from build123d import *

# Parameters (mm, degrees)
EXTRUDE_1_DEPTH      = 40
FILLET_1_R           = 8
SKETCH_9_R           = 6
CUT_EXTRUDE_7_DEPTH  = 172.172427686
SKETCH_10_R          = 6
CUT_EXTRUDE_14_DEPTH = 172.172427686


with BuildPart() as part:
    # 草图8 → 凸台-拉伸1 (new, symmetric)
    with BuildSketch(Plane.XY):
        Polygon((0, 0), (140, 0), (140, 12), (12, 12), (12, 90), (0, 90), align=None)
    extrude(amount=EXTRUDE_1_DEPTH, both=True)

    # 圆角1
    fillet_1_edges = [part.edges().sort_by_distance(p)[0] for p in [
        (76, 12, 40),
        (12, 51, -40),
    ]]
    fillet(fillet_1_edges, radius=FILLET_1_R)

    # 草图9 → 切除-拉伸7 (cut, through all)
    with BuildSketch(Plane(origin=(0, 0, 0), x_dir=(1, 0, 0), z_dir=(0, 1, 0))):
        with Locations(Location((40, 6, 0), (0, 0, 90))):
            Circle(SKETCH_9_R)
    extrude(amount=CUT_EXTRUDE_7_DEPTH, mode=Mode.SUBTRACT)

    # 草图10 → 切除-拉伸14 (cut, through all)
    with BuildSketch(Plane(origin=(0, 0, 0), x_dir=(1, 0, 0), z_dir=(0, 1, 0))):
        with Locations(Location((120, 6, 0), (0, 0, 90))):
            Circle(SKETCH_10_R)
    extrude(amount=CUT_EXTRUDE_14_DEPTH, mode=Mode.SUBTRACT)


solid = part.part
The listing builds one solid part. Answer for the finished solid, in the listing's coordinates (mm). A direction names the side the tool comes from. Coordinates: 2 decimals unless noted, no trailing zeros. Loops run counter-clockwise (first coordinate to the right, second up) from the corner with the lowest first, then second, coordinate; pieces in that order, holes last. Notation, with made-up numbers: (53.5, 30.5) -> (92.5, 30.5) arc R27 ccw to (92.5, 53.5) -> close; hole circle Ø8 at (27.25, 20). An arc over 180 degrees is marked (long way). Answer in a Markdown table with one row per item. Add a question column.
1. The part is cut by section A-A, the plane z = -6. Write down the section's boundary in (x, y).
2. The part is cut by section B-B, the plane x = 120. Write down the section's boundary in (y, z).
3. For faces 4 (the cylindrical face through (9.719, 51.546, -37.594)), 5 (the cylindrical face through (75.104, 9.719, 37.594)), 6 (the flat face through (6, 90, 1)), determine the directions among +Z, -Z, +X, -X, +Y, -Y from which every point of the face is accessible in a straight line to the end or side of a thin tool.
4. The part is cut by section C-C, the plane y = 6. Write down the section's boundary in (x, z).
5. The part is cut by section D-D, the plane z = -23. Write down the section's boundary in (x, y), then the cut area to 3 significant figures.
6. Flat-ended cylindrical pins translate along their axes: P1, Ø12, axis at x = 95, z = -9.5, coming from the +Y side; P2, Ø6, axis at y = 22.5, z = -7.5, coming from the +X side. Find the tip coordinate at first contact, or state that the pin passes through.
7. Consider line 1 (X direction, y = 9.25, z = -6); line 2 (X direction, y = 63.5, z = 33.5). Determine where each line is inside the solid, lowest interval first. Write a range as [from, to].
8. Determine the mould class of faces 1 (the flat face through (140, 6, 1)), 2 (the cylindrical face through (45.857, 5.916, -4.699)), 3 (the flat face through (7, 32, 40)) for opening direction X: +X half, -X half, draft (parallel to the pull), parting line (faces both ways), or undercut.
Answer below:
| question | item | result |
|---|---|---|
| 1 | outline | (0, 0) -> (34, 0) -> (34, 12) -> (12, 12) -> (12, 90) -> (0, 90) -> close; (46, 0) -> (114, 0) -> (114, 12) -> (46, 12) -> close; (126, 0) -> (140, 0) -> (140, 12) -> (126, 12) -> close |
| 2 | outline | (0, -40) -> (12, -40) -> (12, -12) -> (0, -12) -> close; (0, 0) -> (12, 0) -> (12, 32) arc R8 ccw to (4, 40) -> (0, 40) -> close |
| 3 | face 4 | -Z, +X, +Y |
| 3 | face 5 | +Z, +X, +Y |
| 3 | face 6 | +Z, -Z, +X, -X, +Y |
| 4 | outline | (0, -40) -> (140, -40) -> (140, 39.75) -> (12, 39.75) -> (12, 40) -> (0, 40) -> close; hole circle Ø12 at (40, -6); hole circle Ø12 at (120, -6) |
| 5 | outline | (0, 0) -> (140, 0) -> (140, 12) -> (12, 12) -> (12, 90) -> (0, 90) -> close |
| 5 | area | 2,620 mm2 |
| 6 | P1 | y = 12 |
| 6 | P2 | x = 12 |
| 7 | line 1 | [0, 34], [46, 114], [126, 140] |
| 7 | line 2 | [0, 12] |
| 8 | face 1 | +X half |
| 8 | face 2 | undercut |
| 8 | face 3 | draft |
